Geometry: final body of the model. Coordinates: model frame, mm. A direction names the side the tool comes from. Round coordinates to 2 decimals unless told otherwise and drop trailing zeros. Loops run counter-clockwise (first coordinate to the right, second up) from the corner with the lowest first, then second, coordinate; pieces in that order, holes last. Notation, with made-up numbers: (37.5, 15.5) - (57.5, 15.5) arc R19 cw to (57.5, 48.5) - close; hole circle Ø11 at (78, -14). An arc over 180 degrees is marked (long way). Answer as CSV lines item,"result".
Autodesk Fusion 360 part; units mm, degrees
sketch "Sketch1" plane through (0, 0, 0) normal (0, 0, 1) x (1, 0, 0)
  line L0 (10.1, -17.15) -> (-10.1, -17.15)
  line L1 (-10.1, -17.15) -> (-10.1, 17.15)
  line L2 (-10.1, 17.15) -> (10.1, 17.15)
  line L3 (10.1, 17.15) -> (10.1, -17.15)
  line L4 (10.1, -17.15) -> (-10.1, 17.15) construction
  line L5 (-10.1, -17.15) -> (10.1, 17.15) construction
  line L6 (11.7, 18.75) -> (-11.7, 18.75)
  line L7 (-11.7, 18.75) -> (-11.7, -18.75)
  line L8 (-11.7, -18.75) -> (11.7, -18.75)
  line L9 (11.7, -18.75) -> (11.7, 18.75)
  line L10 (11.7, 18.75) -> (-11.7, -18.75) construction
  line L11 (-11.7, 18.75) -> (11.7, -18.75) construction
  dimension "d1" = 20.2
  dimension "d2" = 34.3
  dimension "d4" = 1.6
  dimension "d5" = 1.6
extrude "Extrude1" add sketch "Sketch1" along normal blind 7
sketch "Sketch2" plane through (0, 0, 0) normal (0, 0, -1) x (1, 0, 0)
  line L0 (10.1, -17.15) -> (-10.1, -17.15)
  line L1 (-10.1, -17.15) -> (-10.1, 17.15)
  line L2 (-10.1, 17.15) -> (10.1, 17.15)
  line L3 (10.1, 17.15) -> (10.1, -17.15)
  line L4 (11.7, -18.75) -> (11.7, 18.75)
  line L5 (11.7, 18.75) -> (-11.7, 18.75)
  line L6 (-11.7, 18.75) -> (-11.7, -18.75)
  line L7 (-11.7, -18.75) -> (11.7, -18.75)
  line L8 (-11.7, 18.75) -> (11.7, 18.75)
  line L9 (11.7, 18.75) -> (11.7, -18.75)
  line L10 (11.7, -18.75) -> (-11.7, -18.75)
  line L11 (-11.7, -18.75) -> (-11.7, 18.75)
extrude "Extrude2" add sketch "Sketch2" along normal blind 1.4 contours L0 L1 L2 L3 | L4 L5 L6 L7 L8 L9 L10 L11
sketch "Sketch3" plane through (0, -18.75, 0) normal (0, -1, 0) x (1, 0, 0)
  line L0 (11.7, -1.4) -> (11.7, 7)
  line L1 (11.7, 7) -> (-11.7, 7)
  line L2 (-11.7, 7) -> (-11.7, -1.4)
  line L3 (-11.7, -1.4) -> (11.7, -1.4)
  line L4 (-5.52, 7) -> (4.08, 7)
  line L5 (4.08, 7) -> (4.08, 4.6)
  line L6 (4.08, 4.6) -> (-5.52, 4.6)
  line L7 (-5.52, 4.6) -> (-5.52, 7)
  dimension "d10" = 6
  dimension "d11" = 6.18
  dimension "d14" = 9.6
extrude "Extrude3" cut sketch "Sketch3" against normal up to surface (1.6 mm away) contours L1 L4 L5 L6 L7
fillet "Fillet1" radius 1.3 2 edges at (-5.52, -17.95, 4.6) (4.08, -17.95, 4.6)
sketch "Sketch4" plane through (-11.7, 0, 0) normal (-1, 0, 0) x (0, -1, 0)
  line L0 (18.75, -1.4) -> (18.75, 7)
  line L1 (18.75, 7) -> (-18.75, 7)
  line L2 (-18.75, 7) -> (-18.75, -1.4)
  line L3 (-18.75, -1.4) -> (18.75, -1.4)
  line L4 (10.55, 6.65) -> (15.55, 6.65)
  line L5 (15.55, 6.65) -> (15.55, 5.45)
  line L6 (15.55, 5.45) -> (10.55, 5.45)
  line L7 (10.55, 5.45) -> (10.55, 6.65)
  dimension "d17" = 3.2
  dimension "d18" = 5
  dimension "d19" = 1.2
  dimension "d22" = 0.35
extrude "Extrude4" cut sketch "Sketch4" against normal up to surface (1.6 mm away) contours L4 L5 L6 L7
fillet "Fillet2" radius 0.15 4 edges at (-11.7, -13.05, 5.45) (-11.7, -10.55, 6.05) (-11.7, -13.05, 6.65) (-11.7, -15.55, 6.05)
sketch "Sketch5" plane through (0, 0, 7) normal (0, 0, 1) x (-1, 0, 0)
  line L0 (-4.08, 17.15) -> (-4.08, 18.75)
  line L1 (-4.08, 18.75) -> (-11.7, 18.75)
  line L2 (-11.7, 18.75) -> (-11.7, -18.75)
  line L3 (-11.7, -18.75) -> (11.7, -18.75)
  line L4 (11.7, -18.75) -> (11.7, 18.75)
  line L5 (11.7, 18.75) -> (5.52, 18.75)
  line L6 (5.52, 18.75) -> (5.52, 17.15)
  line L7 (5.52, 17.15) -> (10.1, 17.15)
  line L8 (10.1, 17.15) -> (10.1, -17.15)
  line L9 (10.1, -17.15) -> (-10.1, -17.15)
  line L10 (-10.1, -17.15) -> (-10.1, 17.15)
  line L11 (-10.1, 17.15) -> (-4.08, 17.15)
  line L12 (10.9, -17.95) -> (-10.9, -17.95)
  line L13 (-10.9, -17.95) -> (-10.9, 17.95)
  line L14 (-10.9, 17.95) -> (10.9, 17.95)
  line L15 (10.9, 17.95) -> (10.9, -17.95)
  dimension "d26" = 0.8
  dimension "d27" = 0.8
  dimension "d28" = 0.8
  dimension "d29" = 0.8
extrude "Extrude5" add sketch "Sketch5" along normal blind 1.5 contours L0 L6 L7 L8 L9 L10 L11 L12 L13 L14 L15
sketch "Sketch7" plane through (10.9, 0, 0) normal (1, 0, 0) x (0, 1, 0)
  line L0 (-17.95, 7) -> (17.95, 7)
  line L1 (17.95, 7) -> (17.95, 8.5)
  line L2 (17.95, 8.5) -> (-17.95, 8.5)
  line L3 (-17.95, 8.5) -> (-17.95, 7)
  line L4 (-17.95, 8.5) -> (17.95, 7) construction
  line L5 (17.95, 8.5) -> (-17.95, 7) construction
  line L6 (0, 7.75) -> (-14.5, 7.75) construction
  line L7 (7.5, 7.45) -> (-7.5, 7.45)
  line L8 (-7.5, 7.45) -> (-7.5, 8.05)
  line L9 (-7.5, 8.05) -> (7.5, 8.05)
  line L10 (7.5, 8.05) -> (7.5, 7.45)
  line L11 (7.5, 7.45) -> (-7.5, 8.05) construction
  line L12 (-7.5, 7.45) -> (7.5, 8.05) construction
  point P0 (0, 7.75)
  dimension "d32" = 15
  dimension "d33" = 0.6
ref_plane "WorkPlane1" through (0, 0, 7.75) normal (1, 0, 0) x (0, 1, 0)
extrude "Extrude6" cut sketch "Sketch7" against normal blind 0.45 contours L7 L8 L9 L10
fillet "Fillet5" radius 0.2 4 edges at (10.675, -7.5, 7.45) (10.675, -7.5, 8.05) (10.675, 7.5, 7.45) (10.675, 7.5, 8.05)
fillet "Fillet6" radius 0.2 8 edges at (10.9, -7.4414, 7.5086) (10.9, 0, 7.45) (10.9, 7.4414, 7.5086) (10.9, 7.5, 7.75) (10.9, 7.4414, 7.9914) (10.9, 0, 8.05) (10.9, -7.4414, 7.9914) (10.9, -7.5, 7.75)
mirror "Mirror2" about plane through (0, 0, 7.75) normal (1, 0, 0) of "Extrude6"
fillet "Fillet7" radius 0.2 4 edges at (-10.675, 7.5, 7.45) (-10.675, 7.5, 8.05) (-10.675, -7.5, 7.45) (-10.675, -7.5, 8.05)
fillet "Fillet8" radius 0.2 8 edges at (-10.9, -7.4414, 7.9914) (-10.9, -7.5, 7.75) (-10.9, -7.4414, 7.5086) (-10.9, 0, 7.45) (-10.9, 7.4414, 7.5086) (-10.9, 7.5, 7.75) (-10.9, 7.4414, 7.9914) (-10.9, 0, 8.05)
fillet "Fillet9" radius 0.5 8 edges at (-11.7, 18.75, 2.8) (-11.7, -18.75, 2.8) (-11.7, 0, -1.4) (0, -18.75, -1.4) (11.7, -18.75, 2.8) (11.7, 0, -1.4) (11.7, 18.75, 2.8) (0, 18.75, -1.4)
sketch "Sketch8" plane through (0, 17.15, 0) normal (0, -1, 0) x (1, 0, 0)
  line L0 (-10.1, 0) -> (10.1, 0)
  line L1 (10.1, 0) -> (10.1, 8.5)
  line L2 (10.1, 8.5) -> (-10.1, 8.5)
  line L3 (-10.1, 8.5) -> (-10.1, 0)
  line L4 (4, 6.5) -> (5.5, 6.5)
  line L5 (5.5, 6.5) -> (5.5, 5.5)
  line L6 (5.5, 5.5) -> (4, 5.5)
  line L7 (4, 5.5) -> (4, 6.5)
  dimension "d55" = 4.6
  dimension "d56" = 1
  dimension "d57" = 1.5
  dimension "d58" = 2
extrude "Extrude7" cut sketch "Sketch8" against normal up to surface (1.6 mm away) contours L4 L5 L6 L7
fillet "Fillet10" radius 0.3 4 edges at (5.5, 17.95, 5.5) (5.5, 17.95, 6.5) (4, 17.95, 6.5) (4, 17.95, 5.5)
equation "case_thickness = 1.6 mm"
equation "d4 = case_thickness"
equation "d5 = case_thickness"
equation "d8 = case_thickness - 0.2 mm"
equation "d11 = 4.58 mm + case_thickness"
equation "lock_rim = 0.8 mm"
equation "d26 = lock_rim"
equation "d27 = lock_rim"
equation "d28 = lock_rim"
equation "d29 = lock_rim"
equation "d43 = clip_roundness"
equation "d45 = clip_roundness"
equation "clip_roundness = 0.2 mm"
equation "d50 = clip_roundness"
equation "d52 = clip_roundness"
(1) Access query for faces 4 (the face through (-11, -15.55, 6)), 5 (the face through (0, 0, 0)), 6 (the face through (-5.52, -17.8, 6.9)), 7 (the face through (5, 18, 5.5)). Directions: +Z, -Z, +X, -X, +Y, -Y. A direction counts if a zero-diameter tool reaches every point of the face in a straight line with its end or side. Return the directions, or none.
Findings below:
face 4,"-X"
face 5,"+Z"
face 6,"+Z, -Y"
face 7,"+Y"
(2) Material intervals for line 1 along X through (y, z) = (13, 6.5); line 2 along X through (y, z) = (-2, 7.75); line 3 along Y through (x, z) = (-3.5, 4.5), sorted ascending.
Findings below:
line 1,"-11.7 to -10.1, 10.1 to 11.7"
line 2,"-10.45 to -10.1, 10.1 to 10.45"
line 3,"-18.75 to -17.15, 17.15 to 18.75"
(3) Pin query (flat end, axial travel): P1, Ø5, axis at x = 7, y = 14, coming from the +Z side; P2, Ø0.8, axis at x = -1.5, y = -18.5, coming from the +Z side; P3, Ø1.2, axis at y = -2.5, z = 8, coming from the -X side. Return the tip coordinate at first contact, or that it passes through.
Findings below:
P1,"z = 0"
P2,"z = 4.6"
P3,"x = -10.9"
(4) Section A-A (y = -12). Output: boundary loops of the cut face in (x, z), and give its area (3 significant figures).
Findings below:
outline,"(-11.7, -0.9) arc R0.5 ccw to (-11.2, -1.4) - (11.2, -1.4) arc R0.5 ccw to (11.7, -0.9) - (11.7, 7) - (10.9, 7) - (10.9, 8.5) - (10.1, 8.5) - (10.1, 0) - (-10.1, 0) - (-10.1, 5.45) - (-11.55, 5.45) arc R0.15 ccw to (-11.7, 5.3) - close; (-11.7, 6.8) arc R0.15 ccw to (-11.55, 6.65) - (-10.1, 6.65) - (-10.1, 8.5) - (-10.9, 8.5) - (-10.9, 7) - (-11.7, 7) - close"
area,"55.5 mm2"
(5) Draft query along X for faces 1 (the face through (10.5, 2.6, 8.5)), 2 (the face through (-11.7, 0, 3)), 3 (the face through (4.08, -17.8, 6.9)). Return one class per face: pulls with the +X half, pulls with the -X half, needs draft (parallel to the pull), parting line crosses it, or undercut.
Findings below:
face 1,"needs draft"
face 2,"pulls with the -X half"
face 3,"undercut"
(6) Section D-D (y = 3). Output: boundary loops of the cut face in (x, z).
Findings below:
outline,"(-11.7, -0.9) arc R0.5 ccw to (-11.2, -1.4) - (11.2, -1.4) arc R0.5 ccw to (11.7, -0.9) - (11.7, 7) - (10.9, 7) - (10.9, 7.25) arc R0.2 ccw to (10.7, 7.45) - (10.45, 7.45) - (10.45, 8.05) - (10.7, 8.05) arc R0.2 ccw to (10.9, 8.25) - (10.9, 8.5) - (10.1, 8.5) - (10.1, 0) - (-10.1, 0) - (-10.1, 8.5) - (-10.9, 8.5) - (-10.9, 8.25) arc R0.2 ccw to (-10.7, 8.05) - (-10.45, 8.05) - (-10.45, 7.45) - (-10.7, 7.45) arc R0.2 ccw to (-10.9, 7.25) - (-10.9, 7) - (-11.7, 7) - close"
(7) Section C-C (x = -8). Output: boundary loops of the cut face in (y, z), and give its area (3 significant figures).
Findings below:
outline,"(-18.75, -0.9) arc R0.5 ccw to (-18.25, -1.4) - (18.25, -1.4) arc R0.5 ccw to (18.75, -0.9) - (18.75, 7) - (17.95, 7) - (17.95, 8.5) - (17.15, 8.5) - (17.15, 0) - (-17.15, 0) - (-17.15, 8.5) - (-17.95, 8.5) - (-17.95, 7) - (-18.75, 7) - close"
area,"77.2 mm2"
(8) Section B-B (z = 1.25). Output: boundary loops of the cut face in (x, y).
Findings below:
outline,"(-11.7, -18.25) arc R0.5 ccw to (-11.2, -18.75) - (11.2, -18.75) arc R0.5 ccw to (11.7, -18.25) - (11.7, 18.25) arc R0.5 ccw to (11.2, 18.75) - (-11.2, 18.75) arc R0.5 ccw to (-11.7, 18.25) - close; hole (-10.1, -17.15) - (10.1, -17.15) - (10.1, 17.15) - (-10.1, 17.15) - close"
